Drawing for the job (mm, zero at the part's lowest x, y, z). A direction names the side the tool comes from. Round coordinates to 2 decimals unless told otherwise and drop trailing zeros. Loops run counter-clockwise (first coordinate to the right, second up) from the corner with the lowest first, then second, coordinate; pieces in that order, holes last. Notation, with made-up numbers: M -16,-9.75 L -2,-9.75 A8 ccw -2,4.25 Z; hole C 33.25,37 d4. An arc over 180 degrees is marked long. Put each result on its own line as item: value. Start each with the question number.
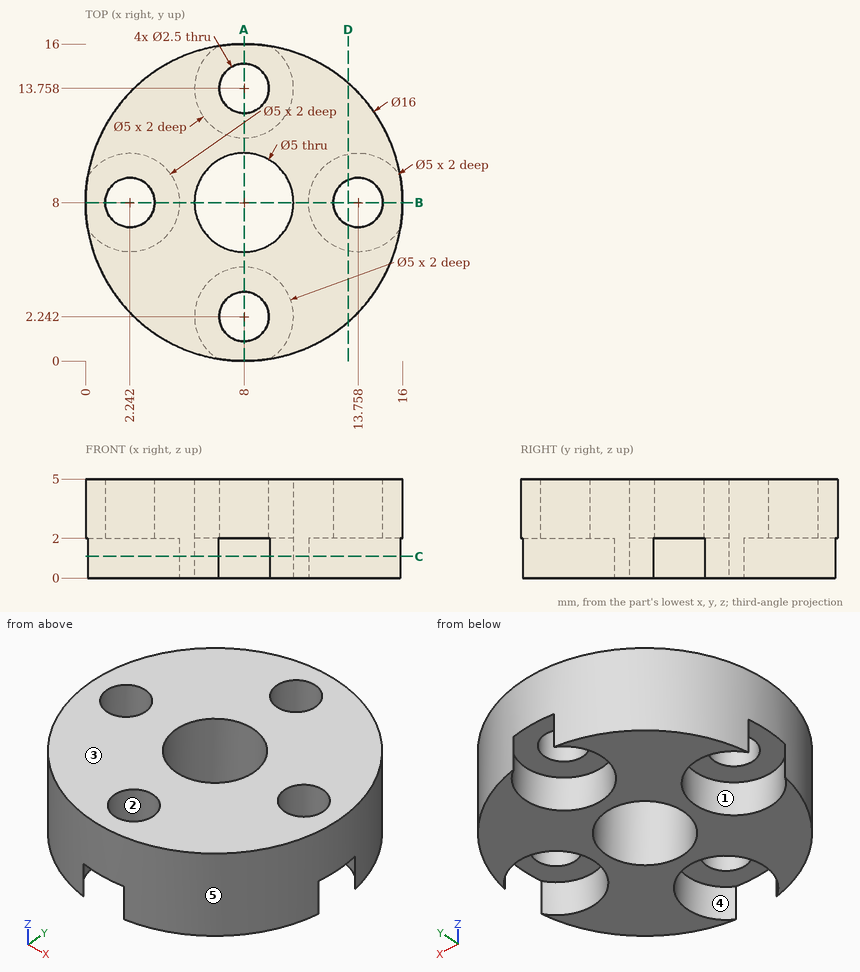
1. Which spindle directions (+Z, -Z, +X, -X, +Y, -Y) get a long thin tool onto all of the face, cutting with end or side? Do the marked faces 1 and 2. Say none if no direction does.
2. Mould opens along X. For the marked faces 3, 4 and 5 say: released by +X, released by -X, zero draft, split by the parting line, or undercut.
3. Drop flat-ended pins along their axis: pin 1 (2 mm diameter, centred on x = 12.5, z = 0.5, fed in from -Y); pin 2 (1 mm diameter, centred on y = 4.5, z = 1, fed in from +X); pin 3 (1 mm diameter, centred on y = 14, z = 1, fed in from +X). Give the stop position or say it passes through.
4. Cut at C-C, the plane z = 1.1. Give the cut face in (x, y).
5. Cut at D-D, the plane x = 13.25. Give the cut face in (y, z).
6. Cut at A-A, the plane x = 8. Give the cut face in (y, z).
7. Wall check: L1, parallel to Y at x = 8, z = 1.25; L2, parallel to Y at x = 8.25, z = 4.05; L3, parallel to X at y = 7.25, z = 2.25 (1 decimal). Give the ranges that are in metal, low to high.
Results list:
1. face 1: -Z
1. face 2: +Z, -Z
2. face 3: zero draft
2. face 4: undercut
2. face 5: split by the parting line
3. pin 1: stops at y = 0.81
3. pin 2: stops at x = 15.42
3. pin 3: stops at x = 13.81
4. outline: M 0.11,6.7 A8 ccw 6.7,0.11 A2.5 cw long 9.3,0.11 A8 ccw 15.89,6.7 A2.5 cw long 15.89,9.3 A8 ccw 9.3,15.89 A2.5 cw long 6.7,15.89 A8 ccw 0.11,9.3 A2.5 cw long Z; hole C 8,8 d5
5. outline: M 1.96,0 L 5.55,0 L 5.55,2 L 6.86,2 L 6.86,5 L 1.96,5 Z; M 9.14,2 L 10.45,2 L 10.45,0 L 14.04,0 L 14.04,5 L 9.14,5 Z
6. outline: M 0,2 L 0.99,2 L 0.99,5 L 0,5 Z; M 3.49,2 L 4.74,2 L 4.74,0 L 5.5,0 L 5.5,5 L 3.49,5 Z; M 10.5,0 L 11.26,0 L 11.26,2 L 12.51,2 L 12.51,5 L 10.5,5 Z; M 15.01,2 L 16,2 L 16,5 L 15.01,5 Z
7. L1: y = 4.74 to 5.5, 10.5 to 11.26
7. L2: y = 0 to 1.02, 3.47 to 5.51, 10.49 to 12.53, 14.98 to 16
7. L3: x = 0 to 1.2, 3.2 to 5.6, 10.4 to 12.8, 14.8 to 16
